Print and shaded views of the part. All mm, measured from the part's lowest x, y and z. A direction names the side the tool comes from. Coordinates: 2 decimals unless noted, no trailing zeros. Order: outer loops, then holes, each group sorted by start corner. A loop starts at its lowest first (then second) coordinate and runs counter-clockwise, first axis right, second up. Notation, with made-up numbers: (-10, -28.75) - (28, -28.75) arc R23 cw to (28, 4.25) - close; hole circle Ø4 at (42, 85). An arc over 180 degrees is marked (long way). Write each question's results on one line, items separated by ' | '.
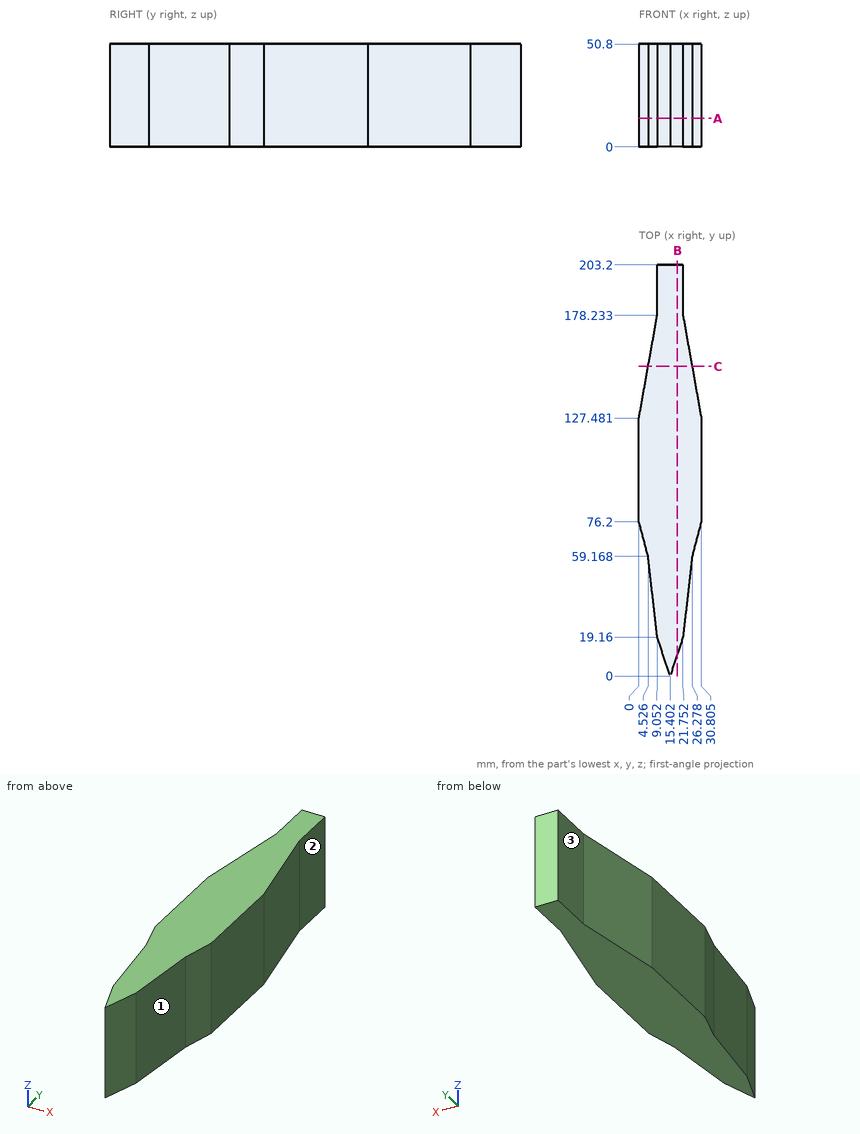
1. Drop a flat-ended pin along its axis: pin 1 Ø10 at (y, z) = (46, 7.5) entering from -X. Give the stop position or say it passes through.
Solved:
pin 1: stops at x = 5.45
2. Tool access for the marked faces 1, 2 and 3: list every direction of +Z, -Z, +X, -X, +Y, -Y with a clear straight run to the whole face (end or side of a thin tool).
Solved:
face 1: +Z, -Z, +X, -Y | face 2: +Z, -Z, +X, +Y | face 3: +Z, -Z, -X, +Y
3. Band-saw the part on A-A on z = 14. Give the cut face in (x, y) (1 decimal).
Solved:
outline: (0, 76.2) - (4.5, 59.2) - (9.1, 19.2) - (15.4, 0) - (21.8, 19.2) - (26.3, 59.2) - (30.8, 76.2) - (30.8, 127.5) - (21.8, 178.2) - (21.8, 203.2) - (9.1, 203.2) - (9.1, 178.2) - (0, 127.5) - close
4. Probe line 1 (X direction, y = 178.5, z = 35.5); line 2 (X direction, y = 143.5, z = 20). List the from-to ranges inside material, lowest first.
Solved:
line 1: x = 9.05 to 21.75 | line 2: x = 2.86 to 27.95
5. Band-saw the part on C-C on y = 153. Give the cut face in (x, z).
Solved:
outline: (4.55, 0) - (26.25, 0) - (26.25, 50.8) - (4.55, 50.8) - close
6. Band-saw the part on B-B on x = 19. Give the cut face in (y, z) (1 decimal).
Solved:
outline: (10.9, 0) - (203.2, 0) - (203.2, 50.8) - (10.9, 50.8) - close
